```python
from build123d import *

# Parameters (mm, degrees)
SKETCH1_R           = 90
BOSS_EXTRUDE1_DEPTH = 23
SKETCH2_R           = 12.5
CUT_EXTRUDE1_DEPTH  = 130.340635533
SKETCH3_R           = 10
CUT_EXTRUDE2_DEPTH  = 15.19384
CIRPATTERN1_START   = 7.806159758
CIRPATTERN1_DEPTH   = 15.193840242


# Read off the part's stored shape, not the designer's step: CirPattern1
with BuildPart() as part:
    # Sketch1 → Boss-Extrude1 (new body)
    with BuildSketch(Plane(origin=(0, 0, 0), x_dir=(1, 0, 0), z_dir=(0, 1, 0))):
        with Locations(Location((0, 0, 0), (0, 0, 270))):
            Circle(SKETCH1_R)
    extrude(amount=BOSS_EXTRUDE1_DEPTH)

    # Sketch2 → Cut-Extrude1 (cut, through all)
    with BuildSketch(Plane(origin=(0, 0, 0), x_dir=(1, 0, 0), z_dir=(0, 1, 0))):
        with Locations(Location((0, 0, 0), (0, 0, 270))):
            Circle(SKETCH2_R)
    extrude(amount=CUT_EXTRUDE1_DEPTH, mode=Mode.SUBTRACT)

    # Sketch3 → Cut-Extrude2 (cut)
    with BuildSketch(Plane(origin=(0, 23, 0), x_dir=(1, 0, 0), z_dir=(0, 1, 0))):
        with Locations((-14.407608976, 0)):
            Circle(SKETCH3_R)
    extrude(amount=-CUT_EXTRUDE2_DEPTH, mode=Mode.SUBTRACT)

    # CirPattern1 outline → CirPattern1 (cut)
    with BuildSketch(Plane(origin=(0, 0, 0), x_dir=(1, 0, 0), z_dir=(0, 1, 0)).offset(CIRPATTERN1_START)):
        with BuildLine():
            ThreePointArc((-9.155897999, -8.509966617), (-14.613560203, -9.99787898), (-20.005318096, -8.286474076))
            ThreePointArc((-20.005318096, -8.286474076), (-17.258785819, -17.258785819), (-8.286474075, -20.005318096))
            ThreePointArc((-8.286474075, -20.005318096), (0, -24.407608976), (8.286474075, -20.005318096))
            ThreePointArc((8.286474075, -20.005318096), (17.258785819, -17.258785819), (20.005318096, -8.286474075))
            ThreePointArc((20.005318096, -8.286474075), (24.407608976, 0), (20.005318096, 8.286474075))
            ThreePointArc((20.005318096, 8.286474075), (17.258785819, 17.258785819), (8.286474075, 20.005318096))
            ThreePointArc((8.286474075, 20.005318096), (0, 24.407608976), (-8.286474075, 20.005318096))
            ThreePointArc((-8.286474075, 20.005318096), (-17.258785819, 17.258785819), (-20.005318096, 8.286474075))
            ThreePointArc((-20.005318096, 8.286474075), (-14.613560203, 9.99787898), (-9.155897999, 8.509966617))
            ThreePointArc((-9.155897999, 8.509966617), (12.5, 0), (-9.155897999, -8.509966617))
        make_face()
    extrude(amount=CIRPATTERN1_DEPTH, mode=Mode.SUBTRACT)


solid = part.part
```
The listing builds one solid part. Answer for the finished solid, in the listing's coordinates (mm). A direction names the side the tool comes from. Round coordinates to 2 decimals unless told otherwise and drop trailing zeros. Order: outer loops, then holes, each group sorted by start corner. A loop starts at its lowest first (then second) coordinate and runs counter-clockwise, first axis right, second up. Notation, with made-up numbers: (32, -38) -> (58, -38) arc R5 cw to (58, -29) -> close; hole circle Ø2 at (83, -28.5). An arc over 180 degrees is marked (long way). Answer as CSV lines item,"result".
Q1. A cutting plane is placed at C-C on x = 0. Determine the outline of the cut face in (y, z).
Computed values:
outline,"(0, -90) -> (23, -90) -> (23, -24.41) -> (7.81, -24.41) -> (7.81, -12.5) -> (0, -12.5) -> close; (0, 12.5) -> (7.81, 12.5) -> (7.81, 24.41) -> (23, 24.41) -> (23, 90) -> (0, 90) -> close"
Q2. Consider line 1 (X direction, y = 5.75, z = 0); line 2 (Z direction, x = -15, y = 9.25); line 3 (Y direction, x = 7, z = -15). Determine where each line is inside the solid, lowest interval first. Write a range as from..to.
Computed values:
line 1,"x = -90..-12.5, 12.5..90"
line 2,"z = -88.74..-18.95, 18.95..88.74"
line 3,"y = 0..7.81"
Q3. A cutting plane is placed at D-D on x = -54. Determine the outline of the cut face in (y, z), plus the area to 3 significant figures.
Computed values:
outline,"(0, -72) -> (23, -72) -> (23, 72) -> (0, 72) -> close"
area,"3,310 mm^2"
Q4. Given pin 1 (5 mm diameter, centred on x = -33, y = 12.5, fed in from +Z); pin 2 (6 mm diameter, centred on y = 16, z = -69.5, fed in from -X); pin 3 (8 mm diameter, centred on x = -69.5, y = 14, fed in from -Z); pin 4 (13.5 mm diameter, centred on x = 3.5, z = -4, fed in from +Y), each flat-ended and moving along its own axis, determine where each tip first touches the part or whether it passes through.
Computed values:
pin 1,"stops at z = 84.67"
pin 2,"stops at x = -60.64"
pin 3,"stops at z = -61.72"
pin 4,"passes through"
Q5. For a pull along X with two mould halves and no side action, classify faces 3 (the cylindrical face through (-34.471, 11.339, 83.137)), 4 (the flat face through (-19, 0, -1)), 5 (the cylindrical face through (3.755, 3.848, 11.923)) as +X half, -X half, draft (parallel to the pull), parting line (faces both ways), or undercut.
Computed values:
face 3,"parting line"
face 4,"draft"
face 5,"undercut"
Q6. A cutting plane is placed at A-A on z = 0. Determine the outline of the cut face in (x, y), plus the area to 3 significant figures.
Computed values:
outline,"(-90, 0) -> (-12.5, 0) -> (-12.5, 7.81) -> (-24.41, 7.81) -> (-24.41, 23) -> (-90, 23) -> close; (12.5, 0) -> (90, 0) -> (90, 23) -> (24.41, 23) -> (24.41, 7.81) -> (12.5, 7.81) -> close"
area,"3,200 mm^2"
Q7. Which of the six approach directions +Z, -Z, +X, -X, +Y, -Y give full straight-line access (tool end or side, diameter ignored) to faces 1 (the cylindrical face through (0.137, 15.297, -24.407)), 2 (the flat face through (-19, 23, 19))?
Computed values:
face 1,"+Y"
face 2,"+Z, -Z, +X, -X, +Y"
Q8. A cutting plane is placed at B-B on y = 14. Determine the outline of the cut face in (x, z).
Computed values:
outline,"circle Ø180 at (0, 0); hole (-20.01, -8.29) arc R10 ccw to (-8.29, -20.01) arc R10 ccw to (8.29, -20.01) arc R10 ccw to (20.01, -8.29) arc R10 ccw to (20.01, 8.29) arc R10 ccw to (8.29, 20.01) arc R10 ccw to (-8.29, 20.01) arc R10 ccw to (-20.01, 8.29) arc R10 ccw to start"
